Read the model definition and answer for the solid it produces. Units are mm, in the model's axes. Give positions to 0.01 mm unless a question says otherwise; leave off trailing zeros. Write each loop counter-clockwise with the first axis right and the second up, starting at its lowest first coordinate (ties: lowest second). Pieces come first, ordered by that corner, then holes. Notation, with made-up numbers: M 69,73 L 107,73 A13 cw 107,98 Z; hole C -28.75,-1 d11. An arc over 180 degrees is marked long. Write each question's results on one line, items separated by ' | '. Start each with the question number.
```python
from build123d import *

# Parameters (mm, degrees)
BOSS_EXTRUDE1_DEPTH = 2
FILLET1_R           = 2


with BuildPart() as part:
    # Sketch1 → Boss-Extrude1 (new body)
    with BuildSketch(Plane.XY):
        Polygon((-35, 7), (-45, 2.5), (-95, 2.5), (-103, 0), (-95, -2.5), (-45, -2.5), (-35, -7), (35, -7), (35, 7), align=None)
    extrude(amount=BOSS_EXTRUDE1_DEPTH)

    # Fillet1
    fillet1_edges = [part.edges().sort_by_distance(p)[0] for p in [
        (35, -7, 1),
        (-35, -7, 1),
        (-45, -2.5, 1),
        (-95, -2.5, 1),
        (-95, 2.5, 1),
        (-45, 2.5, 1),
        (-35, 7, 1),
        (35, 7, 1),
    ]]
    fillet(fillet1_edges, radius=FILLET1_R)


solid = part.part
```
Item 1: Given P1, Ø0.6, axis at x = -78.5, z = 1.5, coming from the -Y side; P2, Ø1, axis at x = -73, y = -1, coming from the -Z side; P3, Ø0.6, axis at x = -80, z = 1, coming from the +Y side, each flat-ended and moving along its own axis, determine where each tip first touches the part or whether it passes through.
Item 2: Section B-B, the plane x = -53.5 is taken. Determine the outline of the cut face in (y, z).
Item 3: Section A-A, the plane z = 1.35 is taken. Determine the outline of the cut face in (x, y).
Item 4: Straight lines are drawn through the part: line 1 (Y direction, x = -79, z = 0.15); line 2 (X direction, y = -3, z = 1.7); line 3 (X direction, y = 4.5, z = 0.9). For each, find the intervals that lie inside material, in ascending order.
Worked out:
1) P1: stops at y = -2.5 | P2: stops at z = 0 | P3: stops at y = 2.5
2) outline: M -2.5,0 L 2.5,0 L 2.5,2 L -2.5,2 Z
3) outline: M -103,0 L -95.29,-2.41 A2 ccw -94.69,-2.5 L -45.43,-2.5 A2 cw -44.61,-2.68 L -35.39,-6.82 A2 ccw -34.57,-7 L 33,-7 A2 ccw 35,-5 L 35,5 A2 ccw 33,7 L -34.57,7 A2 ccw -35.39,6.82 L -44.61,2.68 A2 cw -45.43,2.5 L -94.69,2.5 A2 ccw -95.29,2.41 Z
4) line 1: y = -2.5 to 2.5 | line 2: x = -43.89 to 35 | line 3: x = -40.56 to 35
